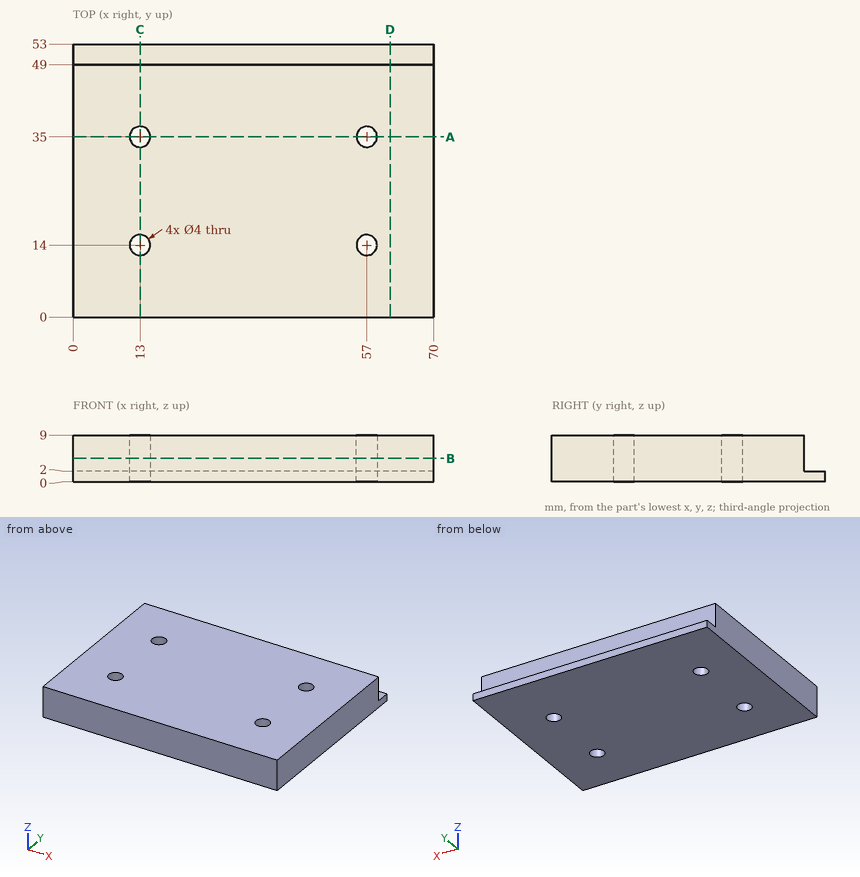
Job drawing, mm, ordinate dimensions from the low corner. One solid piece. Coordinates: 2 decimals unless noted, no trailing zeros. Order: outer loops, then holes, each group sorted by start corner. A loop starts at its lowest first (then second) coordinate and runs counter-clockwise, first axis right, second up. Notation, with made-up numbers: (28, 28) -> (44, 28) arc R22 cw to (44, 49) -> close; hole circle Ø11 at (-6, 61). An arc over 180 degrees is marked (long way). Put each result on its own line as item: value. Start each with the question number.
(1) Band-saw the part on A-A (y = 35). Give the cut face in (x, z).
(2) Band-saw the part on D-D (x = 61.5). Give the cut face in (y, z), then the cut area to 3 significant figures.
(3) Pin check, flat tips, straight feed: pin 1 Ø1.2 at (x, y) = (49, 50) entering from +Z; pin 2 Ø3.5 at (x, z) = (50, 6) entering from +Y. Stop position of each tip, or through.
(4) Band-saw the part on B-B (z = 4.5). Give the cut face in (x, y).
(5) Probe line 1 along Y through (x, z) = (57, 3.5); line 2 along Y through (x, z) = (57.5, 8.5); line 3 along X through (y, z) = (12.5, 8.5). List the from-to ranges inside material, lowest first. Write a range as [from, to].
(6) Band-saw the part on C-C (x = 13). Give the cut face in (y, z), then the cut area to 3 significant figures.
Determined:
1. outline: (0, 0) -> (11, 0) -> (11, 9) -> (0, 9) -> close; (15, 0) -> (55, 0) -> (55, 9) -> (15, 9) -> close; (59, 0) -> (70, 0) -> (70, 9) -> (59, 9) -> close
2. outline: (0, 0) -> (53, 0) -> (53, 2) -> (49, 2) -> (49, 9) -> (0, 9) -> close
2. area: 449 mm²
3. pin 1: stops at z = 2
3. pin 2: stops at y = 49
4. outline: (0, 0) -> (70, 0) -> (70, 49) -> (0, 49) -> close; hole circle Ø4 at (13, 14); hole circle Ø4 at (13, 35); hole circle Ø4 at (57, 14); hole circle Ø4 at (57, 35)
5. line 1: y = [0, 12], [16, 33], [37, 49]
5. line 2: y = [0, 12.06], [15.94, 33.06], [36.94, 49]
5. line 3: x = [0, 11.68], [14.32, 55.68], [58.32, 70]
6. outline: (0, 0) -> (12, 0) -> (12, 9) -> (0, 9) -> close; (16, 0) -> (33, 0) -> (33, 9) -> (16, 9) -> close; (37, 0) -> (53, 0) -> (53, 2) -> (49, 2) -> (49, 9) -> (37, 9) -> close
6. area: 377 mm²
